Source: CAD feature listing. Evaluate the final solid. Frame: model axes, mm. A direction names the side the tool comes from. Coordinates: 2 decimals unless noted, no trailing zeros. Order: outer loops, then holes, each group sorted by start corner. A loop starts at its lowest first (then second) coordinate and runs counter-clockwise, first axis right, second up.
Autodesk Inventor part; units mm, degrees
ref_plane "YZ Plane" through (0, 0, 0) normal (1, 0, 0) x (0, 1, 0)
ref_plane "XZ Plane" through (0, 0, 0) normal (0, 1, 0) x (-1, 0, 0)
ref_plane "XY Plane" through (0, 0, 0) normal (0, 0, 1) x (1, 0, 0)
sketch "Boceto1" plane through (0, 0, 0) normal (1, 0, 0) x (0, 1, 0)
  line L0 (0, 0) -> (15, 0)
  line L1 (15, 0) -> (15, -33)
  line L2 (15, -33) -> (0, -33)
  circle A0 centre (7.5, -8.5) radius 1.5
  circle A1 centre (7.5, -24.5) radius 1.5
  circle A2 centre (7.5, -16.5) radius 1.5
  line L3 (0, -16.5) -> (-3, -16.5)
  line L4 (-3, -16.5) -> (-3, -8.25)
  line L5 (-3, -24.75) -> (-3, -33)
  line L6 (-3, -33) -> (0, -33)
  line L7 (0, -8.25) -> (-3, -8.25)
  line L8 (-3, -24.75) -> (0, -24.75)
  line L9 (0, 0) -> (0, -8.25)
  line L10 (0, -16.5) -> (0, -24.75)
  dimension "d0" = 33
  dimension "d4" = 3
  dimension "d5" = 3
  dimension "d6" = 3
  dimension "d8" = 8.25
  dimension "d9" = 8.25
  dimension "d10" = 8.25
  dimension "d11" = 8.25
extrude "Extrusión1" add sketch "Boceto1" along normal blind 3
properties part number "muñeca6"
1. Section query C-C on z = -25.5. Return loops of the section in (x, y).
Findings:
outline: (0, -3) - (3, -3) - (3, 6.38) - (0, 6.38) - close; (0, 8.62) - (3, 8.62) - (3, 15) - (0, 15) - close
2. Access query for faces 5 (the face through (1, -2, -24.75)), 6 (the face through (1, -1, -8.25)), 7 (the face through (1, 6, -33)). Directions: +Z, -Z, +X, -X, +Y, -Y. A direction counts if a zero-diameter tool reaches every point of the face in a straight line with its end or side. Return the directions, or none.
Findings:
face 5: +X, -X, -Y
face 6: +Z, +X, -X, -Y
face 7: -Z, +X, -X, +Y, -Y
3. Ray query, line 1 (Z direction, x = 1.65, y = 7.5); line 2 (Z direction, x = 0.2, y = 6.25); line 3 (Z direction, x = 1.05, y = -2). Return the intervals inside material, ascending.
Findings:
line 1: z = -33 to -26, -23 to -18, -15 to -10, -7 to 0
line 2: z = -33 to -25.33, -23.67 to -17.33, -15.67 to -9.33, -7.67 to 0
line 3: z = -33 to -24.75, -16.5 to -8.25
4. Pin query (flat end, axial travel): P1, Ø1.5, axis at x = 2, z = -4.5, coming from the -Y side; P2, Ø0.9, axis at x = 1, y = -1, coming from the +Z side. Return the tip coordinate at first contact, or that it passes through.
Findings:
P1: stops at y = 0
P2: stops at z = -8.25
5. Section query A-A on x = 2.6. Return loops of the section in (y, z), plus the area to 3 significant figures.
Findings:
outline: (-3, -33) - (15, -33) - (15, 0) - (0, 0) - (0, -8.25) - (-3, -8.25) - (-3, -16.5) - (0, -16.5) - (0, -24.75) - (-3, -24.75) - close; hole circle Ø3 at (7.5, -24.5); hole circle Ø3 at (7.5, -16.5); hole circle Ø3 at (7.5, -8.5)
area: 523 mm2
6. Draft query along Z for faces 1 (the face through (1, 15, -16)), 2 (the face through (1, 7, 0)), 3 (the face through (1.48, 6.39, -17.51)), 4 (the face through (1.479, 7.305, -25.987)). Return one class per face: released by +Z, released by -Z, zero draft, split by the parting line, or undercut.
Findings:
face 1: zero draft
face 2: released by +Z
face 3: undercut
face 4: undercut
7. Section query B-B on y = 7.5. Return loops of the section in (x, z), plus the area to 3 significant figures.
Findings:
outline: (0, -33) - (3, -33) - (3, -26) - (0, -26) - close; (0, -23) - (3, -23) - (3, -18) - (0, -18) - close; (0, -15) - (3, -15) - (3, -10) - (0, -10) - close; (0, -7) - (3, -7) - (3, 0) - (0, 0) - close
area: 72.0 mm2
8. Section query D-D on z = -3.5. Return loops of the section in (x, y).
Findings:
outline: (0, 0) - (3, 0) - (3, 15) - (0, 15) - close
